```python
from build123d import *

# Parameters (mm, degrees)
F0_W           = 16
F0_H           = 13
F0_R           = 1.65
F1_DEPTH       = 3
F2_R           = 2.2197148543
F3_DEPTH       = 13
F4_R           = 0.585
F5_DEPTH       = 25
F7_DEPTH       = 25
F9_DEPTH       = 13
F10_W          = 7.79368474
F10_H          = 8.6547567695
F11_DEPTH      = 25
F11_DEPTH_BACK = 25


with BuildPart() as f1:
    # F0 (on Top) → F1 (new body)
    with BuildSketch(Plane.XY):
        with Locations((8, 6.5)):
            Rectangle(F0_W, F0_H)
        with Locations((3.1225297134, 2.8979986639)):
            Circle(F0_R, mode=Mode.SUBTRACT)
        with Locations((12.8527397134, 2.8979986639)):
            Circle(F0_R, mode=Mode.SUBTRACT)
        with Locations((3.1225297134, 9.7759086639)):
            Circle(F0_R, mode=Mode.SUBTRACT)
        with Locations((12.8527397134, 9.7759086639)):
            Circle(F0_R, mode=Mode.SUBTRACT)
    extrude(amount=F1_DEPTH)

    # F2 (on face) → F3 (join, through all)
    with BuildSketch(Plane(origin=(0, 13, 0), x_dir=(-1, 0, 0), z_dir=(0, 1, 0))):
        with Locations((-8, 3)):
            Circle(F2_R)
    extrude(amount=-F3_DEPTH)

    # F4 (on face) → F5 (cut)
    with BuildSketch(Plane(origin=(0, 13, 0), x_dir=(-1, 0, 0), z_dir=(0, 1, 0))):
        with Locations((-8, 3)):
            Circle(F4_R)
        Polygon((-8, 0.8955585654), (-9.5511529364, 0), (-6.4488470636, 0), align=None)
    extrude(amount=-F5_DEPTH, mode=Mode.SUBTRACT)

    # F6 (on face) → F7 (cut)
    with BuildSketch(Plane(origin=(0, 13, 0), x_dir=(-1, 0, 0), z_dir=(0, 1, 0))):
        with BuildLine():
            ThreePointArc((-5.7802851457, 3), (-6.4976685136, 1.3659454907), (-8.1861204126, 0.7881018951))
            Line((-8.1861204126, 0.7881018951), (-9.5511529364, 0))
            Line((-9.5511529364, 0), (0, -1.0680041742))
            Line((0, -1.0680041742), (0, 3))
            Line((0, 3), (-5.7802851457, 3))
        make_face()
    extrude(amount=-F7_DEPTH, mode=Mode.SUBTRACT)

    # F8 (on face) → F9 (join, through all)
    with BuildSketch(Plane(origin=(0, 13, 0), x_dir=(-1, 0, 0), z_dir=(0, 1, 0))):
        Polygon((-8, 0.8955585654), (-9.5511529364, 0), (-7.8138795874, 0.7881018951), align=None)
    extrude(amount=-F9_DEPTH)

    # F10 (on face) → F11 (cut, two sides)
    with BuildSketch(Plane.XY.offset(3)) as f11_sk:
        with Locations((6.3228724843, 10.8273783848)):
            Rectangle(F10_W, F10_H)
    extrude(amount=-F11_DEPTH, mode=Mode.SUBTRACT)
    extrude(f11_sk.sketch, amount=F11_DEPTH_BACK, mode=Mode.SUBTRACT)


solid = f1.part
```
Geometry check sheet. Reference: the model listing, model coordinates, mm. A direction names the side the tool comes from. Coordinates: 2 decimals unless noted, no trailing zeros. Order: outer loops, then holes, each group sorted by start corner. A loop starts at its lowest first (then second) coordinate and runs counter-clockwise, first axis right, second up. Notation, with made-up numbers: M 52,-16.75 L 59,-16.75 A26 cw 59,0.25 Z; hole C 56,24 d3. An arc over 180 degrees is marked long. Answer as a JSON object with one key per item and string values.
Q1. Scan lines: line 1 (X direction, y = 5.5, z = 3.05); line 2 (Y direction, x = 14, z = 2.7); line 3 (Z direction, x = 11.25, y = 4.25). Record each from-to range of solid material in increasing order.
Results are:
{"line 1": "x = 5.78 to 7.42, 8.58 to 10.22", "line 2": "y = 0 to 1.71, 4.08 to 8.59, 10.96 to 13", "line 3": "z = 0 to 3"}
Q2. Depth check by flat-ended pin: pin 1 Ø0.9 at (y, z) = (9.5, 2) entering from -X; pin 2 Ø3 at (x, y) = (14, 9) entering from +Z. Enter the tip coordinate at first touch or a pass-through.
Results are:
{"pin 1": "stops at x = 10.22", "pin 2": "stops at z = 3"}
Q3. Cross-section at B-B on y = 2.75. Record the cut outline in (x, z) (3 decimals), and give its area (3 significant figures).
Results are:
{"outline": "M 7.814,0.788 L 9.551,0 L 11.209,0 L 11.209,3 L 10.22,3 A2.22 ccw long Z; M 14.496,0 L 16,0 L 16,3 L 14.496,3 Z; hole C 8,3 d1.17", "area": "24.1 mm²"}
Q4. Cross-section at D-D on z = 1.35. Record the cut outline in (x, y), and give its area (3 significant figures).
Results are:
{"outline": "M 6.52,0 L 16,0 L 16,13 L 10.22,13 L 10.22,6.5 L 6.52,6.5 Z; hole C 12.85,2.9 d3.3; hole C 12.85,9.78 d3.3", "area": "82.1 mm²"}
Q5. Cross-section at A-A on y = 6. Record the cut outline in (x, z) (3 decimals), and give its area (3 significant figures).
Results are:
{"outline": "M 7.814,0.788 L 9.551,0 L 16,0 L 16,3 L 10.22,3 A2.22 ccw long Z; hole C 8,3 d1.17", "area": "34.0 mm²"}
Q6. Release check for a two-part mould opening along Y. For faces 1 (the cylindrical face through (8.584, 3.296, 3.026)), 2 (the cylindrical face through (12.495, 1.287, 1.479)), 3 (the flat face through (7, 6.5, 3)) record: released by +Y, released by -Y, zero draft, split by the parting line, or undercut.
Results are:
{"face 1": "zero draft", "face 2": "undercut", "face 3": "released by +Y"}
Q7. Tool access check on faces 4 (the flat face through (10.22, 10, 2)), 5 (the flat face through (13, 13, 2)), 6 (the flat face through (13, 7, 3)). Record the directions out of +Z, -Z, +X, -X, +Y, -Y that give a thin tool (end or side, any length) a straight path to the whole face; none if there is none.
Results are:
{"face 4": "+Z, -Z, -X, +Y", "face 5": "+Z, -Z, +X, -X, +Y", "face 6": "+Z, +X, +Y, -Y"}
Q8. Cross-section at C-C on x = 8. Record the cut outline in (y, z) (3 decimals), and give its area (3 significant figures).
Results are:
{"outline": "M 0,0.704 L 6.5,0.704 L 6.5,2.415 L 0,2.415 Z; M 0,3.585 L 6.5,3.585 L 6.5,5.22 L 0,5.22 Z", "area": "21.7 mm²"}
